```python
from build123d import *

# Parameters (mm, degrees)
F0_W     = 203.2
F0_H     = 304.8
F1_DEPTH = 12.7
F2_R     = 5.08
F3_W     = 190.5
F3_H     = 292.1
F4_DEPTH = 1.5875
F5_R     = 5.08
F6_R     = 10.16
F7_DEPTH = 25.4


with BuildPart() as f1:
    # F0 (on Top) → F1 (new body)
    with BuildSketch(Plane.XY):
        Rectangle(F0_W, F0_H)
    extrude(amount=F1_DEPTH)

    # F2
    f2_edges = [f1.edges().sort_by_distance(p)[0] for p in [
        (-101.6, 152.4, 6.35),
        (-101.6, -152.4, 6.35),
        (101.6, -152.4, 6.35),
        (101.6, 152.4, 6.35),
    ]]
    fillet(f2_edges, radius=F2_R)

    # F3 (on face) → F4 (cut)
    with BuildSketch(Plane.XY.offset(12.7)):
        Rectangle(F3_W, F3_H)
    extrude(amount=-F4_DEPTH, mode=Mode.SUBTRACT)

    # F5
    f5_edges = [f1.edges().sort_by_distance(p)[0] for p in [
        (95.25, -146.05, 11.90625),
        (-95.25, -146.05, 11.90625),
        (95.25, 146.05, 11.90625),
        (-95.25, 146.05, 11.90625),
    ]]
    fillet(f5_edges, radius=F5_R)

    # F6 (on face) → F7 (join)
    with BuildSketch(Plane(origin=(0, 0, 0), x_dir=(1, 0, 0), z_dir=(0, 0, -1))):
        Circle(F6_R)
    extrude(amount=F7_DEPTH)


solid = f1.part
```
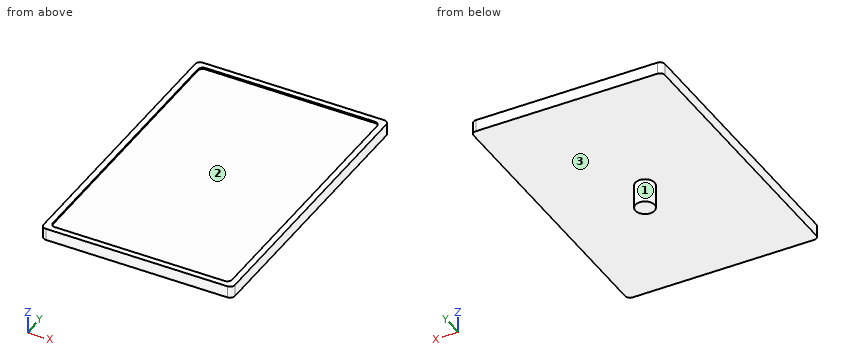
Verification items for the finished model (mm, model axes). Face numbers are marked on the shaded views. Give positions to 0.01 mm unless a question says otherwise; leave off trailing zeros. Order: outer loops, then holes, each group sorted by start corner. A loop starts at its lowest first (then second) coordinate and runs counter-clockwise, first axis right, second up. Notation, with made-up numbers: M 23,57.5 L 47,57.5 A14 cw 47,77.5 Z; hole C 7.5,61 d6. An arc over 180 degrees is marked long. Return JSON: item names as keys, results as strings. Group by question number.
1) Mould release check, pull along Y, two halves, no side actions. Record for the marked faces 1, 2 and 3: pulls with the +Y half, pulls with the -Y half, needs draft (parallel to the pull), parting line crosses it, or undercut.
2) Section check B-B on y = -37.5. Record the cut outline in (x, z), and give its area (3 significant figures).
3) Go/stop test with flat-tipped pins: pin 1 Ø1.5 at (x, y) = (8.5, -105) entering from -Z; pin 2 Ø1 at (y, z) = (1.5, -19.5) entering from +X; pin 3 Ø8 at (x, y) = (-15.5, -30.5) entering from +Z. Record where each tip stops, or that it passes through.
4) Section check C-C on z = -20.5. Record the cut outline in (x, y).
5) Scan lines: line 1 (Z direction, x = -66.5, y = 39.5); line 2 (Y direction, x = -3.5, z = -13); line 3 (Y direction, x = 5.5, z = -13.5). Record each from-to range of solid material in increasing order.
6) Section check A-A on x = -38. Record the cut outline in (y, z), and give its area (3 significant figures).
7) Section check D-D on x = 0. Record the cut outline in (y, z), and give its area (3 significant figures).
Answer block:
{
 "1": {"face 1": "parting line crosses it", "face 2": "undercut", "face 3": "needs draft"},
 "2": {"outline": "M -101.6,0 L 101.6,0 L 101.6,12.7 L 95.25,12.7 L 95.25,11.11 L -95.25,11.11 L -95.25,12.7 L -101.6,12.7 Z", "area": "2,280 mm^2"},
 "3": {"pin 1": "stops at z = 0", "pin 2": "stops at x = 10.11", "pin 3": "stops at z = 11.11"},
 "4": {"outline": "C 0,0 d20.32"},
 "5": {"line 1": "z = 0 to 11.11", "line 2": "y = -9.54 to 9.54", "line 3": "y = -8.54 to 8.54"},
 "6": {"outline": "M -152.4,0 L 152.4,0 L 152.4,12.7 L 146.05,12.7 L 146.05,11.11 L -146.05,11.11 L -146.05,12.7 L -152.4,12.7 Z", "area": "3,410 mm^2"},
 "7": {"outline": "M -152.4,0 L -10.16,0 L -10.16,-25.4 L 10.16,-25.4 L 10.16,0 L 152.4,0 L 152.4,12.7 L 146.05,12.7 L 146.05,11.11 L -146.05,11.11 L -146.05,12.7 L -152.4,12.7 Z", "area": "3,920 mm^2"}
}
